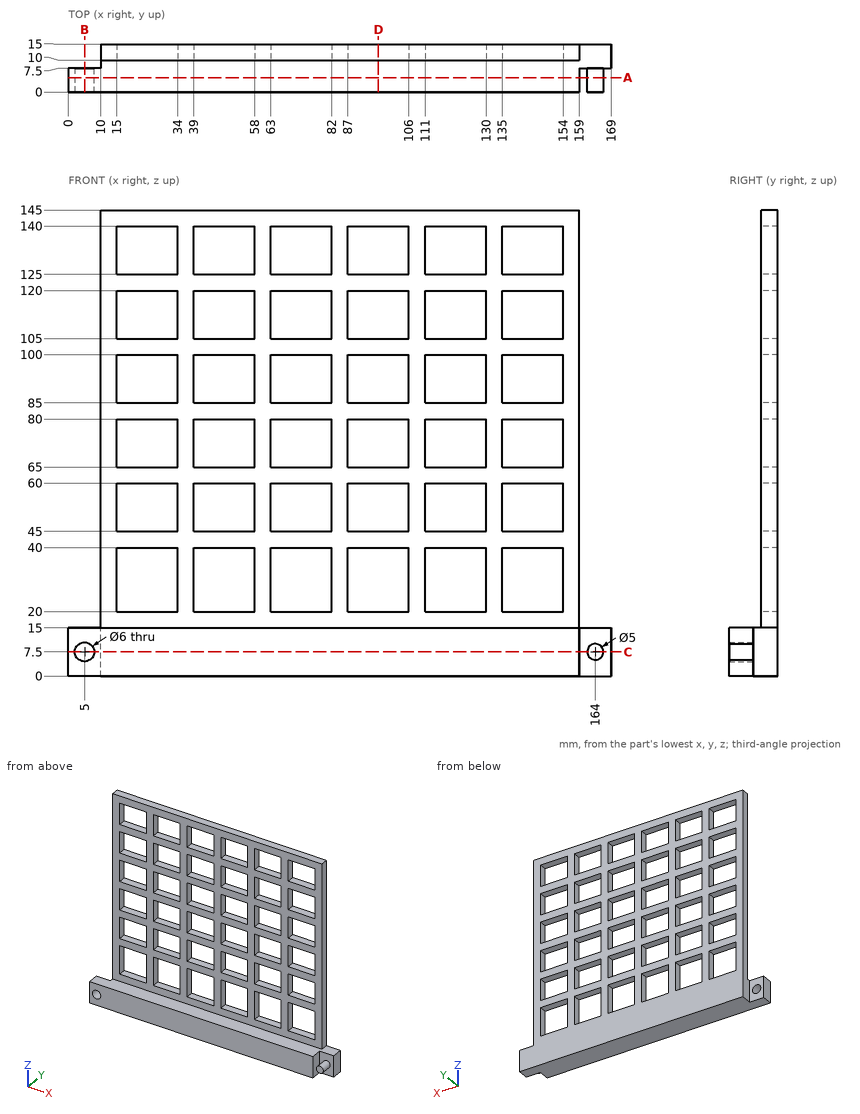
Can you work these out from the drawing? Everything is in mm from the part's minimum corner. Coordinates: 2 decimals unless noted, no trailing zeros. Order: outer loops, then holes, each group sorted by start corner. A loop starts at its lowest first (then second) coordinate and runs counter-clockwise, first axis right, second up. Notation, with made-up numbers: (77, 61) -> (110, 61) arc R21 ccw to (110, 100) -> close; hole circle Ø7 at (-21.75, -1.75). An arc over 180 degrees is marked (long way). Use one line per item in the form item = value.
Q1. Imagine slicing it at B-B, the plane x = 5. List the corners of the cut face in (y, z) for me.
From the geometry:
outline = (0, 0) -> (7.5, 0) -> (7.5, 4.5) -> (0, 4.5) -> close; (0, 10.5) -> (7.5, 10.5) -> (7.5, 15) -> (0, 15) -> close
Q2. Will these pins go through, and if not, where does the flat tip stop? P1, Ø5.5, axis at y = 11.5, z = 115.5, coming from the -X side; P2, Ø5, axis at x = 144, y = 4, coming from the +Z side; P3, Ø5.5, axis at x = 68.5, y = 12, coming from the -Z side; P4, Ø4, axis at y = 13, z = 109.5, coming from the +X side.
From the geometry:
P1 = 10
P2 = 15
P3 = 0
P4 = 159
Q3. I need wall thicknesses on L1, parallel to Z at x = 5, y = 4; L2, parallel to X at y = 5.75, z = 7; L3, parallel to Z at x = 113, y = 3.75. Which ranges of each line are inside material? Lowest first, please.
From the geometry:
L1 = 0 to 4.5, 10.5 to 15
L2 = 0 to 2.04, 7.96 to 159, 161.55 to 166.45
L3 = 0 to 15
Q4. Imagine slicing it at C-C, the plane z = 7.5. List the corners of the cut face in (x, y) for me, then the cut area to 3 significant figures.
From the geometry:
outline = (0, 0) -> (2, 0) -> (2, 7.5) -> (0, 7.5) -> close; (8, 0) -> (159, 0) -> (159, 7.5) -> (161.5, 7.5) -> (161.5, 0) -> (166.5, 0) -> (166.5, 7.5) -> (169, 7.5) -> (169, 15) -> (10, 15) -> (10, 7.5) -> (8, 7.5) -> close
area = 2,380 mm²
Q5. Imagine slicing it at D-D, the plane x = 96.5. Give the number of separate pieces and of enclosed holes in the cut face, then the cut area to 3 significant figures.
From the geometry:
separate_pieces = 7
enclosed_holes = 0
area = 400 mm²
Q6. Imagine slicing it at A-A, the plane y = 4.5. List the corners of the cut face in (x, z) for me, then the cut area to 3 significant figures.
From the geometry:
outline = (0, 0) -> (159, 0) -> (159, 15) -> (0, 15) -> close; circle Ø5 at (164, 7.5); hole circle Ø6 at (5, 7.5)
area = 2,380 mm²
